from build123d import *

# Parameters (mm, degrees)
SKETCH1_R             = 75
BOSS_EXTRUDE1_DEPTH   = 12
SKETCH2_R             = 7.5
CUT_EXTRUDE1_DEPTH    = 107.742681248
SKETCH3_R             = 7.155815761
CUT_EXTRUDE2_DEPTH    = 8.814392
CIRPATTERN1_START     = 3.185607602
CIRPATTERN1_OUTLINE_R = 7.155815761
CIRPATTERN1_DEPTH     = 8.814392398


# Read off the part's stored shape, not the designer's step: CirPattern1
with BuildPart() as part:
    # Sketch1 → Boss-Extrude1 (new body)
    with BuildSketch(Plane(origin=(0, 0, 0), x_dir=(1, 0, 0), z_dir=(0, 1, 0))):
        with Locations(Location((0, 0, 0), (0, 0, 270))):
            Circle(SKETCH1_R)
    extrude(amount=BOSS_EXTRUDE1_DEPTH)

    # Sketch2 → Cut-Extrude1 (cut, through all)
    with BuildSketch(Plane(origin=(0, 0, 0), x_dir=(1, 0, 0), z_dir=(0, 1, 0))):
        with Locations(Location((0, 0, 0), (0, 0, 270))):
            Circle(SKETCH2_R)
    extrude(amount=CUT_EXTRUDE1_DEPTH, mode=Mode.SUBTRACT)

    # Sketch3 → Cut-Extrude2 (cut)
    with BuildSketch(Plane(origin=(0, 12, 0), x_dir=(1, 0, 0), z_dir=(0, 1, 0))):
        with Locations(Location((-28.813602006, 0, 0), (0, 0, 270))):
            Circle(SKETCH3_R)
    extrude(amount=-CUT_EXTRUDE2_DEPTH, mode=Mode.SUBTRACT)

    # CirPattern1 outline → CirPattern1 (cut)
    with BuildSketch(Plane(origin=(0, 0, 0), x_dir=(1, 0, 0), z_dir=(0, 1, 0)).offset(CIRPATTERN1_START)):
        with Locations((-8.903892689, -27.403363946)):
            Circle(CIRPATTERN1_OUTLINE_R)
        with Locations((23.310693692, -16.936210325)):
            Circle(CIRPATTERN1_OUTLINE_R)
        with Locations((23.310693692, 16.936210325)):
            Circle(CIRPATTERN1_OUTLINE_R)
        with Locations((-8.903892689, 27.403363946)):
            Circle(CIRPATTERN1_OUTLINE_R)
    extrude(amount=CIRPATTERN1_DEPTH, mode=Mode.SUBTRACT)


solid = part.part
Build history of the part. All positions in model axes, mm. A direction names the side the tool comes from. Give positions to 0.01 mm unless a question says otherwise; leave off trailing zeros. Write each loop counter-clockwise with the first axis right and the second up, starting at its lowest first coordinate (ties: lowest second). Pieces come first, ordered by that corner, then holes. Notation, with made-up numbers: (-31.5, 60) - (4.5, 60) arc R7 cw to (4.5, 68) - close; hole circle Ø1 at (-23.75, 69). An arc over 180 degrees is marked (long way). Use one line per item in the form item = value. Start each with the question number.
1. Band-saw the part on D-D on x = 22. Write the cut outline in (y, z), plus the area to 3 significant figures.
2. Probe line 1 (X direction, y = 7.5, z = 0); line 2 (Z direction, x = 24, y = 8.5); line 3 (X direction, y = 2.5, z = 0). List the from-to ranges inside material, lowest first. Write a range as [from, to].
3. Band-saw the part on A-A on z = 0. Write the cut outline in (x, y).
4. Band-saw the part on C-C on y = 7. Write the cut outline in (x, z).
5. 3-axis set-ups, long thin cutter, end or side, ignore diameter. For faces 1 (the face through (-16, 0, -1)), 2 (the face through (-21.72, 7.65, -0.93)): which of +Z, -Z, +X, -X, +Y, -Y reach the whole face in a straight line?
6. Drop flat-ended pins along their axis: pin 1 Ø7 at (x, z) = (20.5, -16) entering from +Y; pin 2 Ø2 at (x, y) = (-3, 8) entering from +Z; pin 3 Ø2 at (y, z) = (6, 43) entering from +X. Give the stop position or say it passes through.
7. Band-saw the part on B-B on x = 0. Write the cut outline in (y, z).
8. Two-plate mould, pull along Z, no slides. Class faces 3 (the face through (-9, 3.186, -28)), 4 (the face through (0.33, 5.916, -7.493)), 5 (the face through (-16, 12, -1)), 6 (the face through (-45.636, 5.916, -59.517)): released by +Z, released by -Z, zero draft, split by the parting line, or undercut.
Conclusion:
q1.outline = (0, -71.7) - (12, -71.7) - (12, -23.97) - (3.19, -23.97) - (3.19, -9.9) - (12, -9.9) - (12, 9.9) - (3.19, 9.9) - (3.19, 23.97) - (12, 23.97) - (12, 71.7) - (0, 71.7) - close
q1.area = 1,470 mm²
q2.line_1 = [-75, -35.97], [-21.66, -7.5], [7.5, 75]
q2.line_2 = [-71.06, -24.06], [-9.81, 9.81], [24.06, 71.06]
q2.line_3 = [-75, -7.5], [7.5, 75]
q3.outline = (-75, 0) - (-7.5, 0) - (-7.5, 12) - (-21.66, 12) - (-21.66, 3.19) - (-35.97, 3.19) - (-35.97, 12) - (-75, 12) - close; (7.5, 0) - (75, 0) - (75, 12) - (7.5, 12) - close
q4.outline = circle Ø150 at (0, 0); hole circle Ø14.31 at (-28.81, 0); hole circle Ø14.31 at (-8.9, -27.4); hole circle Ø14.31 at (-8.9, 27.4); hole circle Ø15 at (0, 0); hole circle Ø14.31 at (23.31, -16.94); hole circle Ø14.31 at (23.31, 16.94)
q5.face_1 = +Z, -Z, +X, -X, -Y
q5.face_2 = +Y
q6.pin_1 = 3.19
q6.pin_2 = 74.97
q6.pin_3 = 62.14
q7.outline = (0, -75) - (12, -75) - (12, -7.5) - (0, -7.5) - close; (0, 7.5) - (12, 7.5) - (12, 75) - (0, 75) - close
q8.face_3 = undercut
q8.face_4 = undercut
q8.face_5 = zero draft
q8.face_6 = split by the parting line
